```python
from build123d import *

# Parameters (mm, degrees)
F1_DEPTH = 7
F2_DEPTH = 25


with BuildPart() as f1:
    # F0 (on Top) → F1 (new body)
    with BuildSketch(Plane.XY):
        with BuildLine():
            ThreePointArc((11.1912532195, 8.8289930758), (13.467047778, 4.6726749835), (14.2546577425, 0))
            ThreePointArc((14.2546577425, 0), (13.467047778, -4.6726749835), (11.1912532195, -8.8289930758))
            ThreePointArc((11.1912532195, -8.8289930758), (27.0551814224, -13.467047778), (36.6371641815, 0))
            ThreePointArc((36.6371641815, 0), (27.0551814224, 13.467047778), (11.1912532195, 8.8289930758))
        make_face()
        with BuildLine():
            ThreePointArc((11, 0), (10.5807877336, 3.0078116524), (9.3551034661, 5.7863666613))
            ThreePointArc((9.3551034661, 5.7863666613), (8.1278486965, 0), (9.3551034661, -5.7863666613))
            ThreePointArc((9.3551034661, -5.7863666613), (10.5807877336, -3.0078116524), (11, 0))
        make_face()
        with BuildLine():
            ThreePointArc((-11.1912532195, -8.8289930758), (-14.2546577425, 0), (-11.1912532195, 8.8289930758))
            ThreePointArc((-11.1912532195, 8.8289930758), (-36.6371641815, 0), (-11.1912532195, -8.8289930758))
        make_face()
        with BuildLine():
            ThreePointArc((-8.1278486965, 0), (-8.4380373202, 2.9575409299), (-9.3551034661, 5.7863666613))
            ThreePointArc((-9.3551034661, 5.7863666613), (-11, 0), (-9.3551034661, -5.7863666613))
            ThreePointArc((-9.3551034661, -5.7863666613), (-8.4380373202, -2.9575409299), (-8.1278486965, 0))
        make_face()
        with BuildLine():
            ThreePointArc((9.3551034661, 5.7863666613), (10.1779900284, 7.3651236609), (11.1912532195, 8.8289930758))
            ThreePointArc((11.1912532195, 8.8289930758), (0, 14.2546577425), (-11.1912532195, 8.8289930758))
            ThreePointArc((-11.1912532195, 8.8289930758), (-10.1779900284, 7.3651236609), (-9.3551034661, 5.7863666613))
            ThreePointArc((-9.3551034661, 5.7863666613), (0, 11), (9.3551034661, 5.7863666613))
        make_face()
        with BuildLine():
            ThreePointArc((-11.1912532195, -8.8289930758), (0, -14.2546577425), (11.1912532195, -8.8289930758))
            ThreePointArc((11.1912532195, -8.8289930758), (10.1779900284, -7.3651236609), (9.3551034661, -5.7863666613))
            ThreePointArc((9.3551034661, -5.7863666613), (0, -11), (-9.3551034661, -5.7863666613))
            ThreePointArc((-9.3551034661, -5.7863666613), (-10.1779900284, -7.3651236609), (-11.1912532195, -8.8289930758))
        make_face()
        with BuildLine():
            ThreePointArc((-9.3551034661, 5.7863666613), (-10.1779900284, 7.3651236609), (-11.1912532195, 8.8289930758))
            ThreePointArc((-11.1912532195, 8.8289930758), (-14.2546577425, 0), (-11.1912532195, -8.8289930758))
            ThreePointArc((-11.1912532195, -8.8289930758), (-10.1779900284, -7.3651236609), (-9.3551034661, -5.7863666613))
            ThreePointArc((-9.3551034661, -5.7863666613), (-11, 0), (-9.3551034661, 5.7863666613))
        make_face()
        with BuildLine():
            ThreePointArc((11.1912532195, -8.8289930758), (13.467047778, -4.6726749835), (14.2546577425, 0))
            ThreePointArc((14.2546577425, 0), (13.467047778, 4.6726749835), (11.1912532195, 8.8289930758))
            ThreePointArc((11.1912532195, 8.8289930758), (10.1779900284, 7.3651236609), (9.3551034661, 5.7863666613))
            ThreePointArc((9.3551034661, 5.7863666613), (10.5807877336, 3.0078116524), (11, 0))
            ThreePointArc((11, 0), (10.5807877336, -3.0078116524), (9.3551034661, -5.7863666613))
            ThreePointArc((9.3551034661, -5.7863666613), (10.1779900284, -7.3651236609), (11.1912532195, -8.8289930758))
        make_face()
        with BuildLine():
            ThreePointArc((9.3551034661, -5.7863666613), (8.1278486965, 0), (9.3551034661, 5.7863666613))
            ThreePointArc((9.3551034661, 5.7863666613), (0, 11), (-9.3551034661, 5.7863666613))
            ThreePointArc((-9.3551034661, 5.7863666613), (-8.4380373202, 2.9575409299), (-8.1278486965, 0))
            ThreePointArc((-8.1278486965, 0), (-8.4380373202, -2.9575409299), (-9.3551034661, -5.7863666613))
            ThreePointArc((-9.3551034661, -5.7863666613), (0, -11), (9.3551034661, -5.7863666613))
        make_face()
    extrude(amount=F1_DEPTH)

    # F0 (on Top) → F2 (cut)
    with BuildSketch(Plane.XY):
        with BuildLine():
            ThreePointArc((9.3551034661, -5.7863666613), (8.1278486965, 0), (9.3551034661, 5.7863666613))
            ThreePointArc((9.3551034661, 5.7863666613), (0, 11), (-9.3551034661, 5.7863666613))
            ThreePointArc((-9.3551034661, 5.7863666613), (-8.4380373202, 2.9575409299), (-8.1278486965, 0))
            ThreePointArc((-8.1278486965, 0), (-8.4380373202, -2.9575409299), (-9.3551034661, -5.7863666613))
            ThreePointArc((-9.3551034661, -5.7863666613), (0, -11), (9.3551034661, -5.7863666613))
        make_face()
        with BuildLine():
            ThreePointArc((-8.1278486965, 0), (-8.4380373202, 2.9575409299), (-9.3551034661, 5.7863666613))
            ThreePointArc((-9.3551034661, 5.7863666613), (-11, 0), (-9.3551034661, -5.7863666613))
            ThreePointArc((-9.3551034661, -5.7863666613), (-8.4380373202, -2.9575409299), (-8.1278486965, 0))
        make_face()
        with BuildLine():
            ThreePointArc((11, 0), (10.5807877336, 3.0078116524), (9.3551034661, 5.7863666613))
            ThreePointArc((9.3551034661, 5.7863666613), (8.1278486965, 0), (9.3551034661, -5.7863666613))
            ThreePointArc((9.3551034661, -5.7863666613), (10.5807877336, -3.0078116524), (11, 0))
        make_face()
    extrude(amount=F2_DEPTH, mode=Mode.SUBTRACT)


solid = f1.part
```
Geometry check sheet. Reference: the model listing, model coordinates, mm. Give positions to 0.01 mm unless a question says otherwise; leave off trailing zeros. Order: outer loops, then holes, each group sorted by start corner. A loop starts at its lowest first (then second) coordinate and runs counter-clockwise, first axis right, second up.
1. Section check D-D, the plane x = 26. Enter the section's corners in (y, z).
2. Gauge pin test, flat ends, axial feed: pin 1 Ø2 at (x, y) = (-9, -4) entering from +Z (1 decimal); pin 2 Ø1.5 at (y, z) = (6, 2.5) entering from +X; pin 3 Ø4 at (y, z) = (-5, 2) entering from -X; pin 4 Ø5 at (x, y) = (24.5, -7) entering from -Z. Record the tip position at first contact, or that the pin passes through.
3. Section check C-C, the plane y = -3.5. Enter the section's corners in (x, z).
4. Release check for a two-part mould opening along X. For faces 1 (the face through (8, -9, 7)), 2 (the face through (-0.18, -14.254, 3.451)) record: pulls with the +X half, pulls with the -X half, needs draft (parallel to the pull), parting line crosses it, or undercut.
5. Section check A-A, the plane y = 7.25. Enter the section's corners in (x, z).
6. Section check B-B, the plane z = 5.25. Enter the section's corners in (x, y).
7. Thickness scan on L1, parallel to X at y = -0.5, z = 5; L2, parallel to X at y = -13, z = 5.5; L3, parallel to X at y = -11.25, z = 0.75. Record the ranges inside material, lowest first.
Values follow:
1. outline: (-13.79, 0) - (13.79, 0) - (13.79, 7) - (-13.79, 7) - close
2. pin 1: passes through
2. pin 2: stops at x = 35.64
2. pin 3: stops at x = -36.32
2. pin 4: stops at z = 0
3. outline: (-36.2, 0) - (-10.43, 0) - (-10.43, 7) - (-36.2, 7) - close; (10.43, 0) - (36.2, 0) - (36.2, 7) - (10.43, 7) - close
4. face 1: needs draft
4. face 2: undercut
5. outline: (-34.66, 0) - (-8.27, 0) - (-8.27, 7) - (-34.66, 7) - close; (8.27, 0) - (34.66, 0) - (34.66, 7) - (8.27, 7) - close
6. outline: (-11.19, -8.83) arc R14.25 ccw to (11.19, -8.83) arc R14.25 ccw (long way) to (11.19, 8.83) arc R14.25 ccw to (-11.19, 8.83) arc R14.25 ccw (long way) to start; hole circle Ø22 at (0, 0)
7. L1: x = -36.63 to -10.99, 10.99 to 36.63
7. L2: x = -28.23 to -16.53, -5.85 to 5.85, 16.53 to 28.23
7. L3: x = -31.14 to -13.63, -8.75 to 8.75, 13.63 to 31.14
